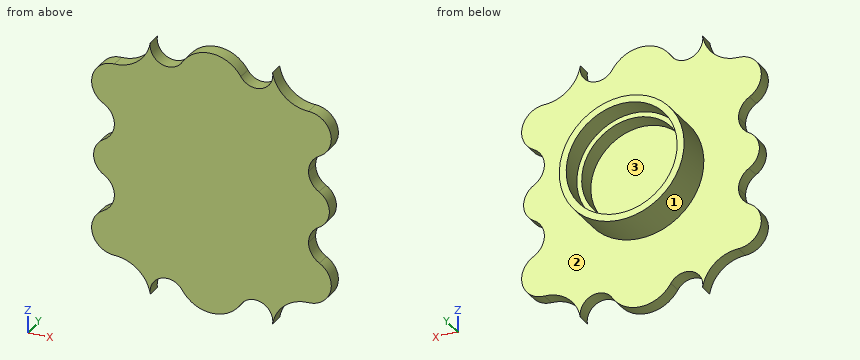
from build123d import *

# Parameters (mm, degrees)
SALIENTE_EXTRUIR1_DEPTH = 10
SALIENTE_EXTRUIR2_DEPTH = 10
CROQUIS3_R              = 40
CROQUIS3_R_2            = 36.5
SALIENTE_EXTRUIR3_DEPTH = 13
CROQUIS4_R              = 45
CROQUIS4_R_2            = 40
SALIENTE_EXTRUIR4_DEPTH = 28


with BuildPart() as part:
    # Croquis1 → Saliente-Extruir1 (new body)
    with BuildSketch(Plane(origin=(0, 0, 0), x_dir=(1, 0, 0), z_dir=(0, 1, 0))):
        with BuildLine():
            Line((-70, -70), (-70, 70))
            ThreePointArc((-70, 70), (-52.983030462, 76.249658661), (-44.055908755, 92.027554074))
            ThreePointArc((-44.055908755, 92.027554074), (-36.156795126, 78.313355526), (-21.147629234, 83.333333333))
            ThreePointArc((-21.147629234, 83.333333333), (0, 95), (21.147629234, 83.333333333))
            ThreePointArc((21.147629234, 83.333333333), (36.156795126, 78.313355526), (44.055908755, 92.027554074))
            ThreePointArc((44.055908755, 92.027554074), (52.983030462, 76.249658661), (70, 70))
            Line((70, 70), (70, -70))
            ThreePointArc((70, -70), (52.983030462, -76.249658661), (44.055908755, -92.027554074))
            ThreePointArc((44.055908755, -92.027554074), (36.156795126, -78.313355526), (21.147629234, -83.333333333))
            ThreePointArc((21.147629234, -83.333333333), (0, -95), (-21.147629234, -83.333333333))
            ThreePointArc((-21.147629234, -83.333333333), (-36.156795126, -78.313355526), (-44.055908755, -92.027554074))
            ThreePointArc((-44.055908755, -92.027554074), (-52.983030462, -76.249658661), (-70, -70))
        make_face()
    extrude(amount=SALIENTE_EXTRUIR1_DEPTH)

    # Croquis2 → Saliente-Extruir2 (add)
    with BuildSketch(Plane(origin=(0, 10, 0), x_dir=(1, 0, 0), z_dir=(0, 1, 0))):
        with BuildLine():
            Line((-70, 25.98076189), (-70, 70))
            ThreePointArc((-70, 70), (-85.909969357, 57.627811916), (-77.837993487, 39.160506523))
            ThreePointArc((-77.837993487, 39.160506523), (-72.107558403, 33.647896498), (-70, 25.98076189))
        make_face()
        with BuildLine():
            ThreePointArc((77.837993487, 39.160506523), (85.909969357, 57.627811916), (70, 70))
            Line((70, 70), (70, 25.98076213))
            ThreePointArc((70, 25.98076213), (72.107558465, 33.647896602), (77.837993487, 39.160506523))
        make_face()
        with BuildLine():
            ThreePointArc((77.5, 12.990381057), (72.009618939, 18.480762121), (70, 25.98076213))
            Line((70, 25.98076213), (70, -25.98076213))
            ThreePointArc((70, -25.98076213), (72.009618939, -18.480762121), (77.5, -12.990381057))
            ThreePointArc((77.5, -12.990381057), (85, 0), (77.5, 12.990381057))
        make_face()
        with BuildLine():
            Line((-70, -25.980762199), (-70, 25.98076189))
            ThreePointArc((-70, 25.98076189), (-72.009618999, 18.480762017), (-77.5, 12.990381057))
            ThreePointArc((-77.5, 12.990381057), (-85, 0), (-77.5, -12.990381057))
            ThreePointArc((-77.5, -12.990381057), (-72.009618922, -18.480762151), (-70, -25.980762199))
        make_face()
        with BuildLine():
            Line((-70, -70), (-70, -25.980762199))
            ThreePointArc((-70, -25.980762199), (-72.107558482, -33.647896631), (-77.837993487, -39.160506523))
            ThreePointArc((-77.837993487, -39.160506523), (-85.909969357, -57.627811916), (-70, -70))
        make_face()
        with BuildLine():
            ThreePointArc((77.837993487, -39.160506523), (72.107558465, -33.647896602), (70, -25.98076213))
            Line((70, -25.98076213), (70, -70))
            ThreePointArc((70, -70), (85.909969357, -57.627811916), (77.837993487, -39.160506523))
        make_face()
    extrude(amount=-SALIENTE_EXTRUIR2_DEPTH)

    # Croquis3 → Saliente-Extruir3 (add)
    with BuildSketch(Plane(origin=(0, 10, 0), x_dir=(1, 0, 0), z_dir=(0, 1, 0))):
        with Locations(Location((0, 0, 0), (0, 0, 90))):
            Circle(CROQUIS3_R)
        with Locations(Location((0, 0, 0), (0, 0, 90))):
            Circle(CROQUIS3_R_2, mode=Mode.SUBTRACT)
    extrude(amount=SALIENTE_EXTRUIR3_DEPTH)

    # Croquis4 → Saliente-Extruir4 (add)
    with BuildSketch(Plane(origin=(0, 10, 0), x_dir=(1, 0, 0), z_dir=(0, 1, 0))):
        with Locations(Location((0, 0, 0), (0, 0, 270))):
            Circle(CROQUIS4_R)
        with Locations(Location((0, 0, 0), (0, 0, 270))):
            Circle(CROQUIS4_R_2, mode=Mode.SUBTRACT)
    extrude(amount=SALIENTE_EXTRUIR4_DEPTH)


solid = part.part
Can you work these out from the model? Positions are in its coordinate system, mm. Face numbers are marked on the shaded views. Give positions to 0.01 mm unless a question says otherwise; leave off trailing zeros. Write each loop counter-clockwise with the first axis right and the second up, starting at its lowest first coordinate (ties: lowest second). Pieces come first, ordered by that corner, then holes. Notation, with made-up numbers: (-21, -34.75) -> (29, -34.75) arc R25 ccw to (29, -6.75) -> close; hole circle Ø8 at (-15.5, 66.25). An arc over 180 degrees is marked (long way). Answer as a JSON object with one key per item and string values. Group by question number.
Item 1: Please list where these lines run through material, in increasing order: line 1 (X direction, y = 33.25, z = 0); line 2 (X direction, y = 20.25, z = 0); line 3 (Y direction, x = 65.5, z = -3). Write a range as [from, to].
Item 2: Suppose I cut it at C-C (y = 33). Please give me the cut outline in (x, z).
Item 3: Suppose I cut it at B-B (x = 0). Please give me the cut outline in (y, z), plus the area to 3 significant figures.
Item 4: I'm going to push flat-ended pins straight in: P1, Ø1.5, axis at y = 13, z = 26.5, coming from the +X side; P2, Ø6, axis at x = -11, y = 14, coming from the +Z side; P3, Ø24, axis at x = -9, z = 5, coming from the +Y side; P4, Ø12, axis at x = 51.5, y = 33.5, coming from the +Z side. Where does each tip first touch, or does it pass through?
Item 5: Suppose I cut it at D-D (z = -60). Please give me the cut outline in (x, y).
Item 6: We'd pull the mould along Z, two halves only. Please class the marked faces 1, 2 and 3: +Z half, -Z half, draft (parallel to the pull), parting line (faces both ways), or undercut.
Item 7: Suppose I cut it at A-A (z = 0). Please give me the cut outline in (x, y), plus the area to 3 significant figures.
Findings:
{
 "1": {"line 1": "x = [-45, -40], [40, 45]", "line 2": "x = [-45, -36.5], [36.5, 45]", "line 3": "y = [0, 10]"},
 "2": {"outline": "circle Ø90 at (0, 0); hole circle Ø80 at (0, 0)"},
 "3": {"outline": "(0, -95) -> (10, -95) -> (10, -45) -> (38, -45) -> (38, -40) -> (23, -40) -> (23, -36.5) -> (10, -36.5) -> (10, 36.5) -> (23, 36.5) -> (23, 40) -> (38, 40) -> (38, 45) -> (10, 45) -> (10, 95) -> (0, 95) -> close", "area": "2,270 mm²"},
 "4": {"P1": "stops at x = 36.9", "P2": "stops at z = 44.28", "P3": "stops at y = 10", "P4": "passes through"},
 "5": {"outline": "(-85.11, 0) -> (85.11, 0) -> (85.11, 10) -> (-85.11, 10) -> close"},
 "6": {"face 1": "parting line", "face 2": "draft", "face 3": "undercut"},
 "7": {"outline": "(-85, 0) -> (85, 0) -> (85, 10) -> (45, 10) -> (45, 38) -> (40, 38) -> (40, 23) -> (36.5, 23) -> (36.5, 10) -> (-36.5, 10) -> (-36.5, 23) -> (-40, 23) -> (-40, 38) -> (-45, 38) -> (-45, 10) -> (-85, 10) -> close", "area": "2,070 mm²"}
}
